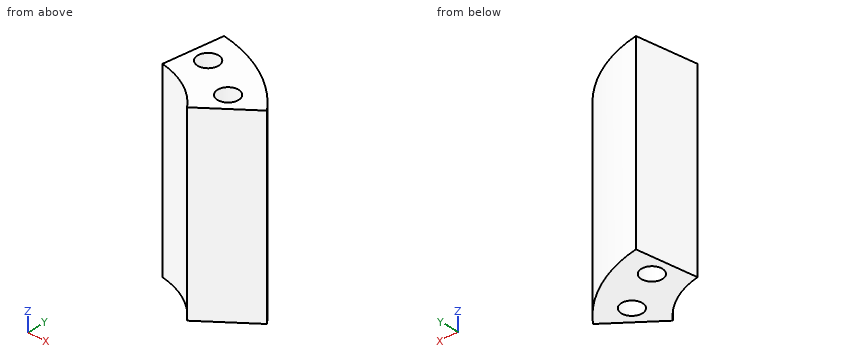
from build123d import *

# Parameters (mm, degrees)
CYLINDER860_R          = 1.5
CYLINDER860_DEPTH      = 60
CYLINDER859_R          = 1.5
CYLINDER859_DEPTH      = 60
BOX336_W               = 20
BOX336_H               = 40
BOX336_DEPTH           = 60
BOX336_PLACEMENT_ANGLE = 22
BOX410_W               = 20
BOX410_H               = 40
BOX410_DEPTH           = 60
BOX410_PLACEMENT_ANGLE = 22
BOX335_W               = 60
BOX335_H               = 40
BOX335_DEPTH           = 60
TUBE037_R              = 20.5
TUBE037_R_2            = 12
TUBE037_DEPTH          = 27
CUT468_PLACEMENT_ANGLE = 30


with BuildPart() as obj1:
    # Cylinder860 → Cylinder860 (new body)
    with BuildSketch(Plane(origin=(-3.5, 16, 0), x_dir=(1, 0, 0), z_dir=(0, 0, 1))):
        Circle(CYLINDER860_R)
    extrude(amount=CYLINDER860_DEPTH)


with BuildPart() as compound565:
    # Cylinder859 → Cylinder859 (new body)
    with BuildSketch(Plane(origin=(3.5, 16, 0), x_dir=(1, 0, 0), z_dir=(0, 0, 1))):
        Circle(CYLINDER859_R)
    extrude(amount=CYLINDER859_DEPTH)

    # Compound565: union obj1
    add(obj1.part)


with BuildPart() as krychle336:
    # Box336 → Box336 (new body)
    with BuildSketch(Plane.XY):
        with Locations((10, 20)):
            Rectangle(BOX336_W, BOX336_H)
    extrude(amount=BOX336_DEPTH)


with BuildPart() as krychle336_1:
    # Box336 placement: moved
    add(krychle336.part.rotate(Axis((0, 0, 0), (0, 0, -1)), BOX336_PLACEMENT_ANGLE))


with BuildPart() as krychle410:
    # Box410 → Box410 (new body)
    with BuildSketch(Plane.XY):
        with Locations((10, 20)):
            Rectangle(BOX410_W, BOX410_H)
    extrude(amount=BOX410_DEPTH)


with BuildPart() as krychle410_1:
    # Box410 placement: moved
    add(krychle410.part.moved(Location((-19.32, -5.18, 0))).rotate(Axis((-19.32, -5.18, 0), (0, 0, 1)), BOX410_PLACEMENT_ANGLE))


with BuildPart() as krychle335:
    # Box335 → Box335 (new body)
    with BuildSketch(Plane(origin=(-30, -35, 0), x_dir=(1, 0, 0), z_dir=(0, 0, 1))):
        with Locations((30, 20)):
            Rectangle(BOX335_W, BOX335_H)
    extrude(amount=BOX335_DEPTH)


with BuildPart() as cut468:
    # Tube037 → Tube037 (new body)
    with BuildSketch(Plane.XY.offset(23)):
        Circle(TUBE037_R)
        Circle(TUBE037_R_2, mode=Mode.SUBTRACT)
    extrude(amount=TUBE037_DEPTH)

    # Cut355: cut Krychle335
    add(krychle335.part, mode=Mode.SUBTRACT)

    # Cut357: cut Krychle410
    add(krychle410_1.part, mode=Mode.SUBTRACT)

    # Cut358: cut Krychle336
    add(krychle336_1.part, mode=Mode.SUBTRACT)

    # Cut468: cut Compound565
    add(compound565.part, mode=Mode.SUBTRACT)


with BuildPart() as cut468_1:
    # Cut468 placement: moved
    add(cut468.part.rotate(Axis((0, 0, 0), (0, 0, -1)), CUT468_PLACEMENT_ANGLE))


solid = cut468_1.part
Design review of the part built by this model. Coordinates are the model's own, in mm. Coordinates: 2 decimals unless noted, no trailing zeros. Loops run counter-clockwise (first coordinate to the right, second up) from the corner with the lowest first, then second, coordinate; pieces in that order, holes last. Notation, with made-up numbers: M 37,-22.5 L 42,-22.5 A26 cw 42,-6.5 Z; hole C -34,-34.5 d11. An arc over 180 degrees is marked long. Answer as CSV lines item,"result".
Item 1: Add section A-A on y = 16.25. State the section outline as (x, z) points.
Answer list:
outline,"M 2.43,23 L 3.61,23 L 3.61,50 L 2.43,50 Z; M 6.32,23 L 12.5,23 L 12.5,50 L 6.32,50 Z"
Item 2: For P1, Ø1.5, axis at x = 7.5, z = 39, coming from the -Y side; P2, Ø3, axis at y = 15, z = 26.5, coming from the -X side, all flat-tipped, find the tip position at first contact; note any pin that passes through.
Answer list:
P1,"y = 8.71"
P2,"x = 2.05"
Item 3: Add section D-D on x = 14.75. State the section outline as (y, z) points, plus the area to 3 significant figures.
Answer list:
outline,"M 11.52,23 L 14.24,23 L 14.24,50 L 11.52,50 Z"
area,"73.2 mm²"
Item 4: Add section B-B on x = 5.75. State the section outline as (y, z) points, plus the area to 3 significant figures.
Answer list:
outline,"M 10.53,23 L 14.33,23 L 14.33,50 L 10.53,50 Z; M 16.89,23 L 19.68,23 L 19.68,50 L 16.89,50 Z"
area,"178 mm²"
Item 5: Add section C-C on z = 27.5. State the section outline as (x, y) points.
Answer list:
outline,"M 1.81,11.86 A12 cw 9.46,7.39 L 16.15,12.62 A20.5 ccw 3,20.28 Z; hole C 4.97,15.61 d3; hole C 11.03,12.11 d3"
Item 6: For probe 1 along Y at (x, z) = (6, 39.75); probe 2 along X at (y, z) = (15, 47.75); probe 3 along Y at (x, z) = (5.5, 30), list the stretches that pass through material, from the lowest coordinate up.
Answer list:
probe 1,"10.39 to 14.52, 16.7 to 19.6"
probe 2,"2.26 to 3.6, 6.34 to 13.97"
probe 3,"10.67 to 14.2, 17.01 to 19.75"
